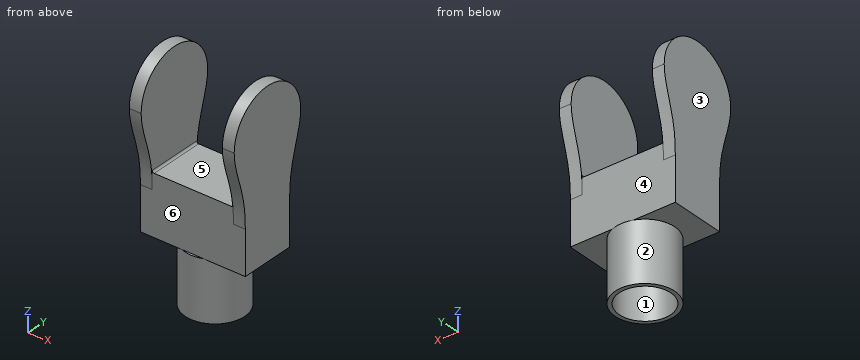
```python
from build123d import *

# Parameters (mm, degrees)
SKETCH1_R           = 15
SKETCH1_R_2         = 13
BOSS_EXTRUDE1_DEPTH = 30
BOSS_EXTRUDE2_START = -3
SKETCH2_R           = 15
BOSS_EXTRUDE2_DEPTH = 3
SKETCH3_W           = 53
SKETCH3_H           = 28
BOSS_EXTRUDE3_DEPTH = 30
BOSS_EXTRUDE5_START = -6
BOSS_EXTRUDE5_DEPTH = 6
FILLET1_R           = 1


# Read off the part's stored shape, not the designer's step: Boss-Extrude5
with BuildPart() as part:
    # Sketch1 → Boss-Extrude1 (new body)
    with BuildSketch(Plane.XY):
        Circle(SKETCH1_R)
        Circle(SKETCH1_R_2, mode=Mode.SUBTRACT)
    extrude(amount=BOSS_EXTRUDE1_DEPTH)

    # Sketch2 → Boss-Extrude2 (add)
    with BuildSketch(Plane.XY.offset(30).offset(BOSS_EXTRUDE2_START)):
        Circle(SKETCH2_R)
    extrude(amount=BOSS_EXTRUDE2_DEPTH)

    # Sketch3 → Boss-Extrude3 (add)
    with BuildSketch(Plane.XY.offset(30)):
        Rectangle(SKETCH3_W, SKETCH3_H)
    extrude(amount=BOSS_EXTRUDE3_DEPTH)

    # Boss-Extrude5 outline → Boss-Extrude5 (add)
    with BuildSketch(Plane(origin=(26.5, 0, 0), x_dir=(0, 0, -1), z_dir=(1, 0, 0)).offset(BOSS_EXTRUDE5_START)):
        with BuildLine():
            Line((-60, 14), (-52.045674019, 14))
            add(Edge.make_bspline(
                [(-52.045674019, 14), (-61.791651738, 14.026298499), (-70.837462314, 14.567622964), (-80.6660896, 21), (-91, 21)],
                knots=[0.062270869, 0.062270869, 0.062270869, 0.062270869, 0.062270869, 1, 1, 1, 1, 1], degree=4))
            ThreePointArc((-91, 21), (-112, 0), (-91, -21))
            add(Edge.make_bspline(
                [(-91, -21), (-80.6660896, -21), (-70.837462314, -14.567622964), (-61.791651738, -14.026298499), (-52.045674019, -14)],
                knots=[0, 0, 0, 0, 0, 0.937729131, 0.937729131, 0.937729131, 0.937729131, 0.937729131], degree=4))
            Line((-52.045674019, -14), (-60, -14))
            Line((-60, -14), (-60, 14))
        make_face()
    boss_extrude5 = extrude(amount=BOSS_EXTRUDE5_DEPTH)

    # Mirror1: Boss-Extrude5 across plane
    add(boss_extrude5.mirror(Plane(origin=(0, 0, 0), x_dir=(0, 0, 1), z_dir=(1, 0, 0))))

    # Fillet1
    fillet1_edges = [part.edges().sort_by_distance(p)[0] for p in [
        (20.5, 0, 60),
        (-20.5, 0, 60),
    ]]
    fillet(fillet1_edges, radius=FILLET1_R)


solid = part.part
```
Design review of the part built by this model. Coordinates are the model's own, in mm. Face numbers are marked on the shaded views. A direction names the side the tool comes from. Coordinates: 2 decimals unless noted, no trailing zeros. Order: outer loops, then holes, each group sorted by start corner. A loop starts at its lowest first (then second) coordinate and runs counter-clockwise, first axis right, second up. Notation, with made-up numbers: (-7, 80) - (11, 80) arc R26 cw to (11, 94) - close; hole circle Ø9 at (25, 55). An arc over 180 degrees is marked (long way). Answer in a Markdown table with one row per item.
(1) Consider section D-D on y = -10. State the section outline as (x, z) points, plus the area to 3 significant figures.
Checked values:
| item | result |
|---|---|
| outline | (-26.5, 30) - (-11.18, 30) - (-11.18, 0) - (-8.31, 0) - (-8.31, 27) - (8.31, 27) - (8.31, 0) - (11.18, 0) - (11.18, 30) - (26.5, 30) - (26.5, 109.47) - (20.5, 109.47) - (20.5, 61) arc R1 cw to (19.5, 60) - (-19.5, 60) arc R1 cw to (-20.5, 61) - (-20.5, 109.47) - (-26.5, 109.47) - close |
| area | 2,410 mm^2 |
(2) Consider section C-C on x = 11.5. State the section outline as (y, z) points, plus the area to 3 significant figures.
Checked values:
| item | result |
|---|---|
| outline | (-14, 30) - (-9.63, 30) - (-9.63, 0) - (-6.06, 0) - (-6.06, 27) - (6.06, 27) - (6.06, 0) - (9.63, 0) - (9.63, 30) - (14, 30) - (14, 60) - (-14, 60) - close |
| area | 1,090 mm^2 |
(3) Clearance check with flat-ended pins moving along their axes: pin 1 (0.8 mm diameter, centred on x = 1.5, y = 14.5, fed in from +Z); pin 2 (6 mm diameter, centred on x = 18, y = 10.5, fed in from -Z); pin 3 (9.5 mm diameter, centred on x = -1, z = 40, fed in from +Y). State where each tip first meets the part, or that it passes through.
Checked values:
| item | result |
|---|---|
| pin 1 | z = 30 |
| pin 2 | z = 30 |
| pin 3 | y = 14 |
(4) For the marked faces 4, 5 and 6, list the 3-axis set-ups (+Z, -Z, +X, -X, +Y, -Y) from which the entire face can be reached by the end or side of a thin tool; tool diameter is ignored.
Checked values:
| item | result |
|---|---|
| face 4 | +Y |
| face 5 | +Z, +Y, -Y |
| face 6 | -Y |
(5) Consider section A-A on x = 0. State the section outline as (y, z) points.
Checked values:
| item | result |
|---|---|
| outline | (-15, 0) - (-13, 0) - (-13, 27) - (13, 27) - (13, 0) - (15, 0) - (15, 30) - (14, 30) - (14, 60) - (-14, 60) - (-14, 30) - (-15, 30) - close |
(6) The part is to be moulded in two halves that separate along X. For the marked faces 1, 2 and 3, say which applies: released by +X, released by -X, zero draft, split by the parting line, or undercut.
Checked values:
| item | result |
|---|---|
| face 1 | undercut |
| face 2 | split by the parting line |
| face 3 | released by -X |
(7) Wall thickness on line 1 along X through (y, z) = (16, 104.5); line 2 along X through (y, z) = (0, 8): over which ranges is each line inside the solid? List them lowest first. Write a range as from..to.
Checked values:
| item | result |
|---|---|
| line 1 | -26.5..-20.5, 20.5..26.5 |
| line 2 | -15..-13, 13..15 |
(8) Consider section B-B on y = 7.5. State the section outline as (x, z) points, plus the area to 3 significant figures.
Checked values:
| item | result |
|---|---|
| outline | (-26.5, 30) - (-12.99, 30) - (-12.99, 0) - (-10.62, 0) - (-10.62, 27) - (10.62, 27) - (10.62, 0) - (12.99, 0) - (12.99, 30) - (26.5, 30) - (26.5, 110.62) - (20.5, 110.62) - (20.5, 61) arc R1 cw to (19.5, 60) - (-19.5, 60) arc R1 cw to (-20.5, 61) - (-20.5, 110.62) - (-26.5, 110.62) - close |
| area | 2,400 mm^2 |
